Could you check a few things on this model? Use its own coordinates, in mm. A direction names the side the tool comes from. Round coordinates to 2 decimals unless told otherwise and drop trailing zeros. Write each loop counter-clockwise with the first axis right and the second up, starting at its lowest first coordinate (ties: lowest second). Pieces come first, ordered by that corner, then holes. Notation, with made-up numbers: M -36.75,82 L 8.25,82 A9 ccw 8.25,99 Z; hole C 63.25,83.25 d9. An arc over 180 degrees is marked long. One line per question, with ' | ' between items. Start each with the question number.
```python
from build123d import *

# Parameters (mm, degrees)
SKETCH_R           = 20.5
PAD_DEPTH          = 3
SKETCH001_R        = 9.75
POCKET_DEPTH       = 3
SKETCH002_R        = 1.65
HOLE_DEPTH         = 25
SKETCH003_R        = 1.65
HOLE001_DEPTH      = 25
PAD001_DEPTH       = 10
POLARPATTERN_COUNT = 3
SKETCH005_R        = 29
PAD002_DEPTH       = 5
SKETCH006_R        = 18.5
POCKET001_DEPTH    = 5
CHAMFER_SIZE       = 1
FILLET_R           = 1
SKETCH007_R        = 1.25
HOLE002_DEPTH      = 25


with BuildPart() as part:
    # Sketch → Pad (new body)
    with BuildSketch(Plane.XY):
        Circle(SKETCH_R)
    extrude(amount=PAD_DEPTH)

    # Sketch001 (on Face3 of Pad) → Pocket (cut)
    with BuildSketch(Plane.XY.offset(3)):
        Circle(SKETCH001_R)
    extrude(amount=-POCKET_DEPTH, mode=Mode.SUBTRACT)

    # Sketch002 (on Face3 of Pocket) → Hole (cut)
    with BuildSketch(Plane.XY.offset(3)):
        with Locations((0, 16.25)):
            Circle(SKETCH002_R)
    extrude(amount=-HOLE_DEPTH, mode=Mode.SUBTRACT)

    # Sketch003 (on Face2 of Hole) → Hole001 (cut)
    with BuildSketch(Plane(origin=(0, 0, 0), x_dir=(1, 0, 0), z_dir=(0, 0, -1))):
        with Locations((-14.072913, 8.125)):
            Circle(SKETCH003_R)
        with Locations((14.072913, 8.125)):
            Circle(SKETCH003_R)
    extrude(amount=-HOLE001_DEPTH, mode=Mode.SUBTRACT)

    # Sketch004 (on Face2 of Hole001) → Pad001 (join)
    with BuildSketch(Plane(origin=(0, 0, 0), x_dir=(1, 0, 0), z_dir=(0, 0, -1))):
        with BuildLine():
            ThreePointArc((11.891571, 14.171822), (0, 18.50666), (-11.891571, 14.171822))
            Line((-13.177146, 15.703911), (-11.891571, 14.171822))
            ThreePointArc((13.177146, 15.703911), (0, 20.506659), (-13.177146, 15.703911))
            Line((11.891571, 14.171822), (13.177146, 15.703911))
        make_face()
    pad001 = extrude(amount=PAD001_DEPTH)

    # PolarPattern: Pad001 ×3 about axis
    polarpattern_axis = Axis((0, 0, 0), (0, 0, -1))
    for i in range(1, POLARPATTERN_COUNT):
        add(pad001.rotate(polarpattern_axis, i * 360 / POLARPATTERN_COUNT))

    # Sketch005 (on Face25 of PolarPattern) → Pad002 (join)
    with BuildSketch(Plane(origin=(0, 0, -10), x_dir=(1, 0, 0), z_dir=(0, 0, -1))):
        Circle(SKETCH005_R)
    extrude(amount=PAD002_DEPTH)

    # Sketch006 (on Face3 of Pad002) → Pocket001 (cut)
    with BuildSketch(Plane(origin=(0, 0, -15), x_dir=(1, 0, 0), z_dir=(0, 0, -1))):
        Circle(SKETCH006_R)
    extrude(amount=-POCKET001_DEPTH, mode=Mode.SUBTRACT)

    # Chamfer
    chamfer_edges = [part.edges().sort_by_distance(p)[0] for p in [
        (15.722913, -8.125, 0),
        (-1.65, 16.25, 0),
        (-12.422913, -8.125, 0),
    ]]
    chamfer(chamfer_edges, length=CHAMFER_SIZE)

    # Fillet
    fillet_edges = [part.edges().sort_by_distance(p)[0] for p in [
        (-20.5, 0, 3),
    ]]
    fillet(fillet_edges, radius=FILLET_R)

    # Sketch007 (on Face33 of Fillet) → Hole002 (cut)
    with BuildSketch(Plane(origin=(0, 0, -15), x_dir=(1, 0, 0), z_dir=(0, 0, -1))):
        with Locations((0, 24)):
            Circle(SKETCH007_R)
        with Locations((-20.78461, -12)):
            Circle(SKETCH007_R)
        with Locations((20.78461, -12)):
            Circle(SKETCH007_R)
    extrude(amount=-HOLE002_DEPTH, mode=Mode.SUBTRACT)


solid = part.part
```
1. Suppose I cut it at D-D (z = -12). Write out the boundary of the cut face in (x, y).
2. Which directions (+Z, -Z, +X, -X, +Y, -Y) give clear straight access to the entire face, cutting with the end or side of a thin tool? Please do faces 1 (the face through (0.2, -20.506, -4.93)), 2 (the face through (6.665, 18.311, -4.93)), 3 (the face through (-12.55, -7.49, 1.99)), 4 (the face through (-4.01, 18.06, -12.54)).
3. Suppose I cut it at B-B (z = -0.75). Write out the boundary of the cut face in (x, y).
4. I need wall thicknesses on line 1 along Y through (x, z) = (0, -13.3); line 2 along X through (y, z) = (12, -13.6); line 3 along Z through (x, y) = (16, 5). Which ranges of each line are inside material? Lowest first, please. Write a range as from..to.
5. I'm going to push flat-ended pins straight in: P1, Ø3, axis at x = 12.5, z = -0.5, coming from the +Y side; P2, Ø2.5, axis at x = -14.07, y = -8.12, coming from the -Z side; P3, Ø5, axis at y = -18.5, z = -1.5, coming from the +X side; P4, Ø6, axis at x = -10.5, z = -1, coming from the +Y side. Where does each tip first touch, or does it pass through?
6. Suppose I cut it at C-C (x = 0). Count the separate pieces of the cut face and the enclosed holes in it, and give its area (3 significant figures).
7. If we mould it in two halves opening along Y, with no side actions, what happens to faces 5 (the face through (19.536, 11.945, -12.535)), 6 (the face through (-0.27, -22.78, -12.54)), 7 (the face through (13.38, 25.73, -12.46)), 8 (the face through (19, 0, -15))? For each: released by +Y, released by -Y, zero draft, split by the parting line, or undercut.
Computed:
1) outline: C 0,0 d58; hole C -20.78,12 d2.5; hole C 0,0 d37; hole C 0,-24 d2.5; hole C 20.78,12 d2.5
2) face 1: +Z, -Y | face 2: +Y | face 3: +Z, -Z | face 4: -Z
3) outline: M -20.19,-3.56 L -18.22,-3.21 A18.48 cw -6.33,17.38 L -7.01,19.26 A20.48 ccw Z; M -13.18,-15.7 A20.48 ccw 13.18,-15.7 L 11.89,-14.17 A18.48 cw -11.89,-14.17 Z; M 6.33,17.38 A18.48 cw 18.22,-3.21 L 20.19,-3.56 A20.48 ccw 7.01,19.26 Z
4) line 1: y = -29..-25.25, -22.75..-18.5, 18.5..29 | line 2: x = -26.4..-22.03, -19.53..-14.08, 14.08..19.53, 22.03..26.4 | line 3: z = 0..3
5) P1: stops at y = 17.3 | P2: passes through | P3: stops at x = 12.82 | P4: stops at y = 19.08
6) separate pieces: 5 | enclosed holes: 0 | area: 166 mm²
7) face 5: undercut | face 6: undercut | face 7: split by the parting line | face 8: zero draft
